from build123d import *

# Parameters (mm, degrees)
F0_W     = 155
F0_H     = 9
F1_DEPTH = 27
F0_H_2   = 13
F2_R     = 4.5
F3_DEPTH = 25


with BuildPart() as f1:
    # F0 (on Top) → F1 (new body)
    with BuildSketch(Plane.XY):
        with Locations((0, 20.5)):
            Rectangle(F0_W, F0_H)
    extrude(amount=F1_DEPTH)



with BuildPart() as f1b:
    # F0 (on Top) → F1, piece 2 (new body)
    with BuildSketch(Plane.XY):
        with Locations((0, -20.5)):
            Rectangle(F0_W, F0_H)
    extrude(amount=F1_DEPTH)


with BuildPart() as f1c:
    # F0 (on Top) → F1, piece 3 (new body)
    with BuildSketch(Plane.XY):
        with Locations((0, 7.5)):
            Rectangle(F0_W, F0_H_2)
    extrude(amount=F1_DEPTH)


with BuildPart() as f1d:
    # F0 (on Top) → F1, piece 4 (new body)
    with BuildSketch(Plane.XY):
        with Locations((0, -7.5)):
            Rectangle(F0_W, F0_H_2)
    extrude(amount=F1_DEPTH)


with BuildPart() as f1_1:
    add(f1.part)

    add(f1b.part)  # F3 merges F1b

    add(f1c.part)  # F3 merges F1c

    add(f1d.part)  # F3 merges F1d
    # F2 (on face) → F3 (join)
    with BuildSketch(Plane.XY.offset(27)):
        Polygon((-77.5, -16), (-77.5, -25), (77.5, -25), (77.5, -16), (77.5, -14), (77.5, -1), (77.5, 1), (77.5, 14), (77.5, 16), (77.5, 25), (-77.5, 25), (-77.5, 16), (-77.5, 14), (-77.5, 1), (-77.5, -1), (-77.5, -14), align=None)
        with Locations((-67.5, -15)):
            Circle(F2_R, mode=Mode.SUBTRACT)
        with Locations((-52.5, -15)):
            Circle(F2_R, mode=Mode.SUBTRACT)
        with Locations((-37.5, -15)):
            Circle(F2_R, mode=Mode.SUBTRACT)
        with Locations((-22.5, -15)):
            Circle(F2_R, mode=Mode.SUBTRACT)
        with Locations((-7.5, -15)):
            Circle(F2_R, mode=Mode.SUBTRACT)
        with Locations((7.5, -15)):
            Circle(F2_R, mode=Mode.SUBTRACT)
        with Locations((22.5, -15)):
            Circle(F2_R, mode=Mode.SUBTRACT)
        with Locations((37.5, -15)):
            Circle(F2_R, mode=Mode.SUBTRACT)
        with Locations((52.5, -15)):
            Circle(F2_R, mode=Mode.SUBTRACT)
        with Locations((67.5, -15)):
            Circle(F2_R, mode=Mode.SUBTRACT)
        with Locations((-67.5, 0)):
            Circle(F2_R, mode=Mode.SUBTRACT)
        with Locations((-52.5, 0)):
            Circle(F2_R, mode=Mode.SUBTRACT)
        with Locations((-37.5, 0)):
            Circle(F2_R, mode=Mode.SUBTRACT)
        with Locations((-22.5, 0)):
            Circle(F2_R, mode=Mode.SUBTRACT)
        with Locations((-7.5, 0)):
            Circle(F2_R, mode=Mode.SUBTRACT)
        with Locations((-67.5, 15)):
            Circle(F2_R, mode=Mode.SUBTRACT)
        with Locations((-52.5, 15)):
            Circle(F2_R, mode=Mode.SUBTRACT)
        with Locations((-37.5, 15)):
            Circle(F2_R, mode=Mode.SUBTRACT)
        with Locations((-22.5, 15)):
            Circle(F2_R, mode=Mode.SUBTRACT)
        with Locations((-7.5, 15)):
            Circle(F2_R, mode=Mode.SUBTRACT)
        with Locations((7.5, 0)):
            Circle(F2_R, mode=Mode.SUBTRACT)
        with Locations((22.5, 0)):
            Circle(F2_R, mode=Mode.SUBTRACT)
        with Locations((37.5, 0)):
            Circle(F2_R, mode=Mode.SUBTRACT)
        with Locations((52.5, 0)):
            Circle(F2_R, mode=Mode.SUBTRACT)
        with Locations((67.5, 0)):
            Circle(F2_R, mode=Mode.SUBTRACT)
        with Locations((7.5, 15)):
            Circle(F2_R, mode=Mode.SUBTRACT)
        with Locations((22.5, 15)):
            Circle(F2_R, mode=Mode.SUBTRACT)
        with Locations((37.5, 15)):
            Circle(F2_R, mode=Mode.SUBTRACT)
        with Locations((52.5, 15)):
            Circle(F2_R, mode=Mode.SUBTRACT)
        with Locations((67.5, 15)):
            Circle(F2_R, mode=Mode.SUBTRACT)
    extrude(amount=F3_DEPTH)


solid = f1_1.part
Check sheet for the modelled part. Datum: model origin and axes. Units: mm. A direction names the side the tool comes from. Give positions to 0.01 mm unless a question says otherwise; leave off trailing zeros. Loops run counter-clockwise (first coordinate to the right, second up) from the corner with the lowest first, then second, coordinate; pieces in that order, holes last. Notation, with made-up numbers: M -31.75,30 L -12.75,30 A19 ccw -12.75,41 Z; hole C -23,-11.75 d8. An arc over 180 degrees is marked long. Answer as a JSON object with one key per item and string values. Group by question number.
Q1. Go/stop test with flat-tipped pins: P1, Ø4, axis at x = 57.5, y = -16.5, coming from the -Z side; P2, Ø0.6, axis at x = -30, y = -14.5, coming from the -Z side; P3, Ø1.8, axis at x = 68, y = -13, coming from the +Z side. Record where each tip stops, or that it passes through.
Q2. Cross-section at B-B on x = 7.5. Record the cut outline in (y, z).
Q3. Cross-section at C-C on z = 4. Record the cut outline in (x, y).
Q4. Access from +Z, -Z, +X, -X, +Y, -Y to the whole of each face (thin tool, end or side, straight path). Record for faces 1 (the flat face through (-1, 16, 13)), 2 (the flat face through (-53, 2, 27)).
Q5. Release check for a two-part mould opening along Y. For faces 3 (the flat face through (-53, -2, 27)), 4 (the flat face through (1, 25, 26)), 5 (the cylindrical face through (-48.208, 16.352, 39.325)) record: released by +Y, released by -Y, zero draft, split by the parting line, or undercut.
Q6. Cross-section at A-A on z = 47.5. Give the number of separate pieces and of enclosed holes in the cut face, then the cut area to 3 significant figures.
Q7. Material ranges on line 1 along Y through (x, z) = (56.5, 14.5); line 2 along Y through (x, z) = (-22.5, 37.75); line 3 along Z through (x, y) = (36, -1.5), recorded low to high. Write a range as [from, to].
Q8. Cross-section at D-D on x = 54.5. Record the cut outline in (y, z), then the cut area to 3 significant figures.
Evaluation:
{
 "1": {"P1": "stops at z = 0", "P2": "stops at z = 27", "P3": "stops at z = 27"},
 "2": {"outline": "M -25,0 L -16,0 L -16,27 L -19.5,27 L -19.5,52 L -25,52 Z; M -14,0 L -1,0 L -1,27 L -4.5,27 L -4.5,52 L -10.5,52 L -10.5,27 L -14,27 Z; M 1,0 L 14,0 L 14,27 L 10.5,27 L 10.5,52 L 4.5,52 L 4.5,27 L 1,27 Z; M 16,0 L 25,0 L 25,52 L 19.5,52 L 19.5,27 L 16,27 Z"},
 "3": {"outline": "M -77.5,-25 L 77.5,-25 L 77.5,-16 L -77.5,-16 Z; M -77.5,-14 L 77.5,-14 L 77.5,-1 L -77.5,-1 Z; M -77.5,1 L 77.5,1 L 77.5,14 L -77.5,14 Z; M -77.5,16 L 77.5,16 L 77.5,25 L -77.5,25 Z"},
 "4": {"face 1": "-Z, +X, -X", "face 2": "+Z"},
 "5": {"face 3": "undercut", "face 4": "released by +Y", "face 5": "undercut"},
 "6": {"separate pieces": "1", "enclosed holes": "30", "area": "5,840 mm2"},
 "7": {"line 1": "y = [-25, -16], [-14, -1], [1, 14], [16, 25]", "line 2": "y = [-25, -19.5], [-10.5, -4.5], [4.5, 10.5], [19.5, 25]", "line 3": "z = [0, 27]"},
 "8": {"outline": "M -25,0 L -16,0 L -16,27 L -19.03,27 L -19.03,52 L -25,52 Z; M -14,0 L -1,0 L -1,27 L -4.03,27 L -4.03,52 L -10.97,52 L -10.97,27 L -14,27 Z; M 1,0 L 14,0 L 14,27 L 10.97,27 L 10.97,52 L 4.03,52 L 4.03,27 L 1,27 Z; M 16,0 L 25,0 L 25,52 L 19.03,52 L 19.03,27 L 16,27 Z", "area": "1,830 mm2"}
}
